Geometry: final body of the model. Coordinates: model frame, mm. A direction names the side the tool comes from. Give positions to 0.01 mm unless a question says otherwise; leave off trailing zeros. Order: outer loops, then holes, each group sorted by start corner. A loop starts at its lowest first (then second) coordinate and runs counter-clockwise, first axis right, second up. Notation, with made-up numbers: M 54,8.25 L 76,8.25 A15 cw 76,14.25 Z; hole C 86.5,27 d1. An arc over 180 degrees is marked long. Use CSV: the item, a comma, the result in double quotes.
```python
from build123d import *

# Parameters (mm, degrees)
BOSS_EXTRUDE1_DEPTH = 25.654
BOSS_EXTRUDE2_DEPTH = 1.27
CUT_EXTRUDE1_REACH  = 65.61
CUT_EXTRUDE2_REACH  = 76.499
SKETCH7_W           = 44.577
SKETCH7_H           = 19.304
CUT_EXTRUDE3_DEPTH  = 8.255
SKETCH8_W           = 18.669
SKETCH8_H           = 26.797
CUT_EXTRUDE4_DEPTH  = 12.7
FILLET2_R           = 2.54
SKETCH9_R           = 2.2098
BOSS_EXTRUDE3_DEPTH = 3.302
CHAMFER1_SIZE       = 1.27


# Some blends are built 0.0001 mm under size
with BuildPart() as part:
    # Sketch2 → Boss-Extrude1 (new body)
    with BuildSketch(Plane.XY):
        with BuildLine():
            Line((-27.305, -23.749), (27.305, -23.749))
            ThreePointArc((27.305, -23.749), (31.076707571, -22.186707571), (32.639, -18.415))
            Line((32.639, -18.415), (32.639, 18.415))
            ThreePointArc((32.639, 18.415), (31.076707571, 22.186707571), (27.305, 23.749))
            Line((27.305, 23.749), (-27.305, 23.749))
            ThreePointArc((-27.305, 23.749), (-31.076707571, 22.186707571), (-32.639, 18.415))
            Line((-32.639, 18.415), (-32.639, -18.415))
            ThreePointArc((-32.639, -18.415), (-31.076707571, -22.186707571), (-27.305, -23.749))
        make_face()
        with BuildLine():
            Line((-27.305, -22.479), (27.305, -22.479))
            ThreePointArc((27.305, -22.479), (30.178681959, -21.288681959), (31.369, -18.415))
            Line((31.369, -18.415), (31.369, 18.415))
            ThreePointArc((31.369, 18.415), (30.178681959, 21.288681959), (27.305, 22.479))
            Line((27.305, 22.479), (-27.305, 22.479))
            ThreePointArc((-27.305, 22.479), (-30.178681959, 21.288681959), (-31.369, 18.415))
            Line((-31.369, 18.415), (-31.369, -18.415))
            ThreePointArc((-31.369, -18.415), (-30.178681959, -21.288681959), (-27.305, -22.479))
        make_face(mode=Mode.SUBTRACT)
    extrude(amount=BOSS_EXTRUDE1_DEPTH)

    # Sketch3 → Boss-Extrude2 (add)
    with BuildSketch(Plane.XY.offset(25.654)):
        with BuildLine():
            Line((-1.778, 23.749), (27.305, 23.749))
            ThreePointArc((27.305, 23.749), (31.076707571, 22.186707571), (32.639, 18.415))
            Line((32.639, 18.415), (32.639, -7.493))
            Line((32.639, -7.493), (32.639, -8.763))
            Line((32.639, -8.763), (-1.778, -8.763))
            Line((-1.778, -8.763), (-1.778, -23.749))
            Line((-1.778, -23.749), (-3.048, -23.749))
            Line((-3.048, -23.749), (-3.048, -8.763))
            Line((-3.048, -8.763), (-32.639, -8.763))
            Line((-32.639, -8.763), (-32.639, -7.493))
            Line((-32.639, -7.493), (-3.048, -7.493))
            Line((-3.048, -7.493), (-3.048, 23.749))
            Line((-3.048, 23.749), (-1.778, 23.749))
        make_face()
        with BuildLine():
            Line((27.559, -7.493), (2.032, -7.493))
            ThreePointArc((2.032, -7.493), (-0.662076836, -6.377076836), (-1.778, -3.683))
            Line((-1.778, -3.683), (-1.778, 18.669))
            ThreePointArc((-1.778, 18.669), (-0.662076836, 21.363076836), (2.032, 22.479))
            Line((2.032, 22.479), (27.305, 22.479))
            ThreePointArc((27.305, 22.479), (30.178681959, 21.288681959), (31.369, 18.415))
            Line((31.369, 18.415), (31.369, -3.683))
            ThreePointArc((31.369, -3.683), (30.253076836, -6.377076836), (27.559, -7.493))
        make_face(mode=Mode.SUBTRACT)
    extrude(amount=BOSS_EXTRUDE2_DEPTH)

    # Sketch5 → Cut-Extrude1 (cut, up to next)
    with BuildSketch(Plane(origin=(0, 23.749, 0), x_dir=(1, 0, 0), z_dir=(0, 1, 0)), mode=Mode.PRIVATE) as cut_extrude1_sk1:
        with BuildLine():
            Line((-21.336, 0), (-21.336, -15.24))
            ThreePointArc((-21.336, -15.24), (-20.592051224, -17.036051224), (-18.796, -17.78))
            Line((-18.796, -17.78), (-12.192, -17.78))
            ThreePointArc((-12.192, -17.78), (-10.395948776, -17.036051224), (-9.652, -15.24))
            Line((-9.652, -15.24), (-9.652, 0))
            Line((-9.652, 0), (-21.336, 0))
        make_face()
    cut_extrude1_tool1 = extrude(cut_extrude1_sk1.sketch, amount=-CUT_EXTRUDE1_REACH, mode=Mode.PRIVATE) & part.part
    add(cut_extrude1_tool1.solids().sort_by_distance((-15.494, 23.749, 8.777566))[0], mode=Mode.SUBTRACT)

    # Sketch6 → Cut-Extrude2 (cut, up to next)
    with BuildSketch(Plane.ZY.offset(32.639), mode=Mode.PRIVATE) as cut_extrude2_sk1:
        with BuildLine():
            Line((8.255, -4.699), (17.145, -4.699))
            ThreePointArc((17.145, -4.699), (18.043025612, -5.070974388), (18.415, -5.969))
            Line((18.415, -5.969), (18.415, -12.319))
            ThreePointArc((18.415, -12.319), (18.043025612, -13.217025612), (17.145, -13.589))
            Line((17.145, -13.589), (8.255, -13.589))
            ThreePointArc((8.255, -13.589), (7.356974388, -13.217025612), (6.985, -12.319))
            Line((6.985, -12.319), (6.985, -5.969))
            ThreePointArc((6.985, -5.969), (7.356974388, -5.070974388), (8.255, -4.699))
        make_face()
    cut_extrude2_tool1 = extrude(cut_extrude2_sk1.sketch, amount=-CUT_EXTRUDE2_REACH, mode=Mode.PRIVATE) & part.part
    add(cut_extrude2_tool1.solids().sort_by_distance((-32.639, -9.144, 12.7))[0], mode=Mode.SUBTRACT)

    # Sketch7 → Cut-Extrude3 (cut)
    with BuildSketch(Plane.XZ.offset(23.749)):
        with Locations((-10.3505, 10.795)):
            Rectangle(SKETCH7_W, SKETCH7_H)
    extrude(amount=-CUT_EXTRUDE3_DEPTH, mode=Mode.SUBTRACT)

    # Sketch8 → Cut-Extrude4 (cut)
    with BuildSketch(Plane(origin=(32.639, 0, 0), x_dir=(0, 0, -1), z_dir=(1, 0, 0))):
        with Locations((-11.43, -10.3505)):
            Rectangle(SKETCH8_W, SKETCH8_H)
    extrude(amount=-CUT_EXTRUDE4_DEPTH, mode=Mode.SUBTRACT)

    # Fillet2
    # the kernel refuses this fillet: 2.54 mm, written as the material it takes off along each edge
    with BuildSketch(Plane(origin=(2.032, 18.669, 25.654), x_dir=(-1, 0, 0), z_dir=(0, -1, 0))) as fillet2_piece_1_section:
        with BuildLine():
            CenterArc((6.009704526, -2.54), FILLET2_R, 90, 60)
            Line((3.81, -1.27), (3.81, 0))
            Line((3.81, 0), (6.009704526, 0))
        make_face()
    fillet2_piece_1 = revolve(axis=Axis((2.032, 18.669, 25.654), (0, 0, -1)), revolution_arc=172.73255531, mode=Mode.PRIVATE)
    fillet2_piece_1 = split(fillet2_piece_1, bisect_by=Plane(origin=(2.032, 22.479, 25.654), z_dir=(0, -1, 0)), keep=Keep.TOP, mode=Mode.PRIVATE)
    add(fillet2_piece_1, mode=Mode.SUBTRACT)
    with BuildSketch(Plane(origin=(2.032, -3.683, 25.654), x_dir=(0, -1, 0), z_dir=(1, 0, 0))) as fillet2_piece_2:
        with BuildLine():
            CenterArc((6.009704526, -2.54), FILLET2_R, 90, 60)
            Line((3.81, -1.27), (3.81, 0))
            Line((3.81, 0), (6.009704526, 0))
        make_face()
    revolve(axis=Axis((2.032, -3.683, 25.654), (0, 0, -1)), revolution_arc=90, mode=Mode.SUBTRACT)
    with BuildSketch(Plane(origin=(27.559, -3.683, 25.654), x_dir=(0.1265009963233053, 0.9919664802447767, 0), z_dir=(-0.9919664802447767, 0.1265009963233053, 0))) as fillet2_piece_3_section:
        with BuildLine():
            CenterArc((6.009704526, -2.54), FILLET2_R, 90, 60)
            Line((3.81, -1.27), (3.81, 0))
            Line((3.81, 0), (6.009704526, 0))
        make_face()
    fillet2_piece_3 = revolve(axis=Axis((27.559, -3.683, 25.654), (0, 0, -1)), revolution_arc=172.73255531, mode=Mode.PRIVATE)
    fillet2_piece_3 = split(fillet2_piece_3, bisect_by=Plane(origin=(31.369, -3.683, 25.654), z_dir=(-1, 0, 0)), keep=Keep.TOP, mode=Mode.PRIVATE)
    add(fillet2_piece_3, mode=Mode.SUBTRACT)
    with BuildSketch(Plane(origin=(27.559, -7.493, 25.654), x_dir=(0, -1, 0), z_dir=(-1, 0, 0))) as fillet2_piece_4:
        with BuildLine():
            CenterArc((2.199704526, 2.54), FILLET2_R, 210, 60)
            Line((0, 1.27), (0, 0))
            Line((0, 0), (2.199704526, 0))
        make_face()
    extrude(amount=25.527, mode=Mode.SUBTRACT)
    with BuildSketch(Plane(origin=(-1.778, -3.683, 25.654), x_dir=(-1, 0, 0), z_dir=(0, 1, 0))) as fillet2_piece_5:
        with BuildLine():
            CenterArc((2.199704526, 2.54), FILLET2_R, 210, 60)
            Line((0, 1.27), (0, 0))
            Line((0, 0), (2.199704526, 0))
        make_face()
    extrude(amount=22.352, mode=Mode.SUBTRACT)

    # Sketch9 → Boss-Extrude3 (add)
    # profile 1 of 2: a face of its own
    with BuildSketch(Plane.XY):
        with BuildLine():
            Line((-29.522086836, 23.2664), (-38.1, 23.2664))
            ThreePointArc((-38.1, 23.2664), (-42.3164, 19.05), (-38.1, 14.8336))
            Line((-38.1, 14.8336), (-32.639, 14.8336))
            Line((-32.639, 14.8336), (-32.639, 18.415))
            ThreePointArc((-32.639, 18.415), (-31.792621708, 21.298193959), (-29.522086836, 23.2664))
        make_face()
        with Locations(Location((-38.1, 19.05, 0), (0, 0, 180))):
            Circle(SKETCH9_R, mode=Mode.SUBTRACT)
    # profile 2 of 2: a face of its own
    with BuildSketch(Plane.XY):
        with BuildLine():
            Line((29.522086836, 23.2664), (38.1, 23.2664))
            ThreePointArc((38.1, 23.2664), (42.3164, 19.05), (38.1, 14.8336))
            Line((38.1, 14.8336), (32.639, 14.8336))
            Line((32.639, 14.8336), (32.639, 18.415))
            ThreePointArc((32.639, 18.415), (31.792621708, 21.298193959), (29.522086836, 23.2664))
        make_face()
        with Locations(Location((38.1, 19.05, 0), (0, 0, 180))):
            Circle(SKETCH9_R, mode=Mode.SUBTRACT)
    extrude(amount=BOSS_EXTRUDE3_DEPTH)

    # Chamfer1
    chamfer1_edges = [part.edges().sort_by_distance(p)[0] for p in [
        (-21.336, 22.479, 7.62),
        (-20.592051224, 22.479, 17.036051224),
        (-15.494, 22.479, 17.78),
        (-10.395948776, 22.479, 17.036051224),
        (-9.652, 22.479, 7.62),
    ]]
    chamfer(chamfer1_edges, length=CHAMFER1_SIZE - 0.0001)  # a hair under: the kernel refuses the full size


solid = part.part
```
1. Section B-B, the plane z = 12.5. Give the number of separate pieces and of enclosed holes in the cut face, plus the area to 3 significant figures.
Answer:
separate pieces,"4"
enclosed holes,"0"
area,"133 mm2"
2. Pin query (flat end, axial travel): pin 1 Ø1 at (x, z) = (-32, 7) entering from -Y; pin 2 Ø10 at (x, y) = (-11, 13.5) entering from -Z; pin 3 Ø1.4 at (y, z) = (-13, 26.5) entering from -X; pin 4 Ø10 at (x, y) = (26, -11) entering from -Z. Return the tip coordinate at first contact, or that it passes through.
Answer:
pin 1,"y = -15.49"
pin 2,"through"
pin 3,"x = -3.05"
pin 4,"z = 25.66"
3. Pull-direction query (X, two-part tool) for faces 1 (the face through (-31.369, 4, 13)), 2 (the face through (32, -13, 2.095)), 3 (the face through (31.035, -22.228, 23.175)); classes: +X half, -X half, draft (parallel to the pull), parting line (faces both ways), or undercut.
Answer:
face 1,"undercut"
face 2,"draft"
face 3,"+X half"
4. Reachability of faces 4 (the face through (0, 22.479, 13)), 5 (the face through (-22, -23, 25.654)), 6 (the face through (35, 14.834, 2)), 7 (the face through (30.147, -21.32, 1.033)) from +Z, -Z, +X, -X, +Y, -Y: full face, straight path, thin tool, end or side. Return the list, or none.
Answer:
face 4,"-Z"
face 5,"+Z, -X, -Y"
face 6,"+Z, -Z, +X, -Y"
face 7,"+Z, -Z"
5. Section A-A, the plane y = 14. Return the cut outline in (x, z), plus the area to 3 significant figures.
Answer:
outline,"M -32.64,0 L -31.37,0 L -31.37,25.65 L -32.64,25.65 Z; M -3.05,25.83 A2.54 ccw -1.78,26.92 L -3.05,26.92 Z; M 31.37,0 L 32.64,0 L 32.64,26.92 L 31.37,26.92 Z"
area,"67.6 mm2"
6. Line query: line 1 (X direction, y = 16.5, z = 24.5); line 2 (Y direction, x = 38.1, z = 1.3); line 3 (X direction, y = 19.05, z = 1.85). Output: solid intervals per line, ascending.
Answer:
line 1,"-32.64 to -31.37, 31.37 to 32.64"
line 2,"14.83 to 16.84, 21.26 to 23.27"
line 3,"-42.32 to -40.31, -35.89 to -31.32, 31.32 to 35.89, 40.31 to 42.32"
